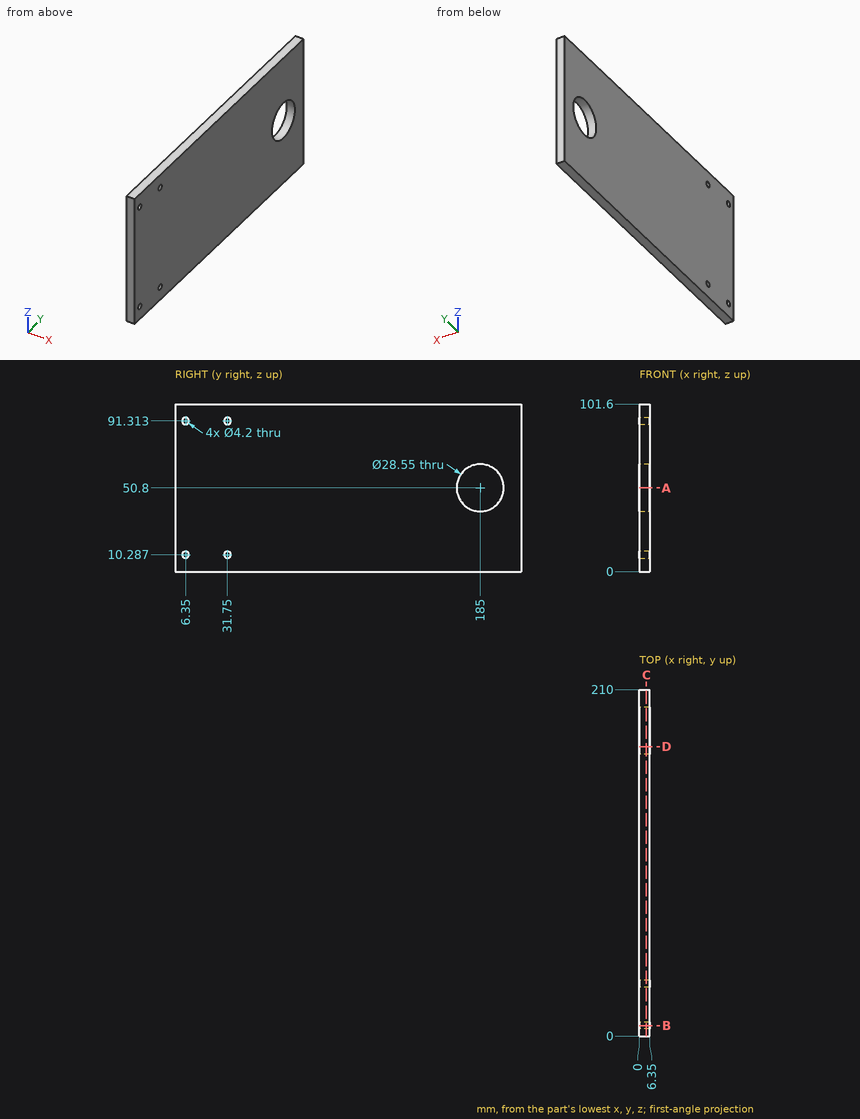
The drawing under review shows one solid part. Ordinate dimensions are in mm from its lowest x, y, z. Round coordinates to 2 decimals unless told otherwise and drop trailing zeros. Loops run counter-clockwise (first coordinate to the right, second up) from the corner with the lowest first, then second, coordinate; pieces in that order, holes last. Notation, with made-up numbers: (49, 86.5) - (63, 86.5) arc R18 ccw to (63, 90.5) - close; hole circle Ø5 at (71, 66). An arc over 180 degrees is marked (long way). Use a Markdown table: item, result. Add a question column.
Q1. Add section C-C (x = 4.25). State the section outline as (y, z) points (3 decimals).
Q2. Add section B-B (y = 6.35). State the section outline as (x, z) points, plus the area to 3 significant figures.
Q3. For probe 1 along Y at (x, z) = (3, 11.5); probe 2 along Y at (x, z) = (4, 50); probe 3 along Y at (x, z) = (1, 45), list the stretches that pass through material, from the lowest coordinate up.
Q4. Add section D-D (y = 175.5). State the section outline as (x, z) points, plus the area to 3 significant figures.
Q5. Add section A-A (z = 50.8). State the section outline as (x, y) points (3 decimals), plus the area to 3 significant figures.
Worked answers:
| question | item | result |
|---|---|---|
| 1 | outline | (0, 0) - (210, 0) - (210, 101.6) - (0, 101.6) - close; hole circle Ø4.2 at (6.35, 10.287); hole circle Ø4.2 at (6.35, 91.313); hole circle Ø4.2 at (31.75, 10.287); hole circle Ø4.2 at (31.75, 91.313); hole circle Ø28.55 at (185, 50.8) |
| 2 | outline | (0, 0) - (6.35, 0) - (6.35, 8.19) - (0, 8.19) - close; (0, 12.39) - (6.35, 12.39) - (6.35, 89.21) - (0, 89.21) - close; (0, 93.41) - (6.35, 93.41) - (6.35, 101.6) - (0, 101.6) - close |
| 2 | area | 592 mm² |
| 3 | probe 1 | 0 to 4.64, 8.06 to 30.04, 33.46 to 210 |
| 3 | probe 2 | 0 to 170.75, 199.25 to 210 |
| 3 | probe 3 | 0 to 171.96, 198.04 to 210 |
| 4 | outline | (0, 0) - (6.35, 0) - (6.35, 40.15) - (0, 40.15) - close; (0, 61.45) - (6.35, 61.45) - (6.35, 101.6) - (0, 101.6) - close |
| 4 | area | 510 mm² |
| 5 | outline | (0, 0) - (6.35, 0) - (6.35, 170.725) - (0, 170.725) - close; (0, 199.275) - (6.35, 199.275) - (6.35, 210) - (0, 210) - close |
| 5 | area | 1,150 mm² |
